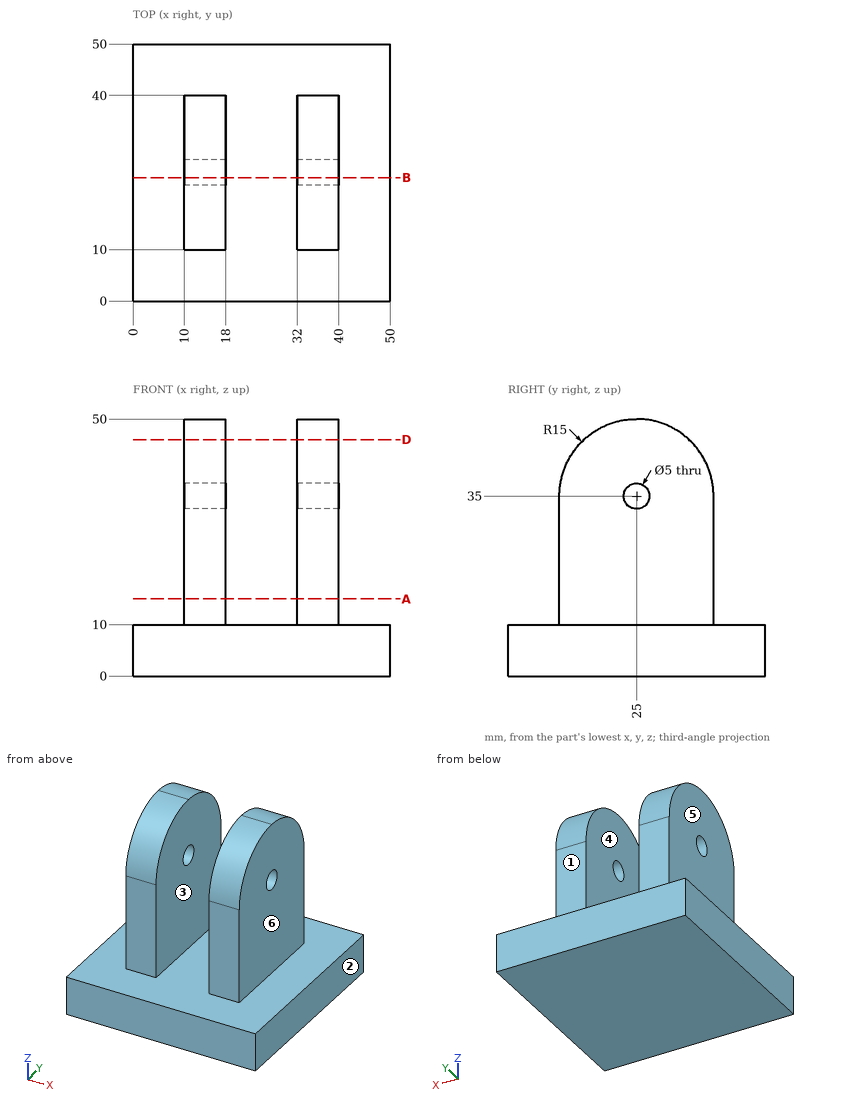
For this review, use the dimensioned drawing (mm, ordinates from the lowest corner) and the shaded views. A direction names the side the tool comes from. Coordinates: 2 decimals unless noted, no trailing zeros. Loops run counter-clockwise (first coordinate to the right, second up) from the corner with the lowest first, then second, coordinate; pieces in that order, holes last. Notation, with made-up numbers: (68.25, 68) -> (99.25, 68) arc R19 ccw to (99.25, 79) -> close; hole circle Ø7 at (-32.75, 37.25). An arc over 180 degrees is marked (long way). Use a Markdown table: item, result. Add a question column.
1. Add section A-A on z = 15. Write out the cut boundary in (x, y), plus the area to 3 significant figures.
2. Clearance check with flat-ended pins moving along their axes: pin 1 Ø6.5 at (x, z) = (12.5, 17.5) entering from +Y; pin 2 Ø2 at (y, z) = (14.5, 25.5) entering from -X; pin 3 Ø9 at (x, z) = (14.5, 26) entering from -Y. State where each tip first meets the part, or that it passes through.
3. Add section D-D on z = 46. Write out the cut boundary in (x, y).
4. Draft analysis for pull direction X (two halves, no side actions). For the marked faces 1, 2 and 3, state which applies: pulls with the +X half, pulls with the -X half, needs draft (parallel to the pull), parting line crosses it, or undercut.
5. Add section B-B on y = 24. Write out the cut boundary in (x, z), plus the area to 3 significant figures.
6. To check wall thickness, follow line 1 (Z direction, x = 15, y = 25); line 2 (X direction, y = 38.5, z = 25.5); line 3 (Z direction, x = 43.5, y = 14.5). State the ranges of each line that lie inside material, in increasing order.
7. Machinability: for the marked faces 4, 5 and 6, which of the approach directions +Z, -Z, +X, -X, +Y, -Y give a long, thin tool a straight path to every point of the face, cutting with its end or side? Answer none if there is none.
Returned:
| question | item | result |
|---|---|---|
| 1 | outline | (10, 10) -> (18, 10) -> (18, 40) -> (10, 40) -> close; (32, 10) -> (40, 10) -> (40, 40) -> (32, 40) -> close |
| 1 | area | 480 mm² |
| 2 | pin 1 | stops at y = 40 |
| 2 | pin 2 | stops at x = 10 |
| 2 | pin 3 | stops at y = 10 |
| 3 | outline | (10, 14.8) -> (18, 14.8) -> (18, 35.2) -> (10, 35.2) -> close; (32, 14.8) -> (40, 14.8) -> (40, 35.2) -> (32, 35.2) -> close |
| 4 | face 1 | needs draft |
| 4 | face 2 | pulls with the +X half |
| 4 | face 3 | undercut |
| 5 | outline | (0, 0) -> (50, 0) -> (50, 10) -> (40, 10) -> (40, 32.71) -> (32, 32.71) -> (32, 10) -> (18, 10) -> (18, 32.71) -> (10, 32.71) -> (10, 10) -> (0, 10) -> close; (10, 37.29) -> (18, 37.29) -> (18, 49.97) -> (10, 49.97) -> close; (32, 37.29) -> (40, 37.29) -> (40, 49.97) -> (32, 49.97) -> close |
| 5 | area | 1,070 mm² |
| 6 | line 1 | z = 0 to 32.5, 37.5 to 50 |
| 6 | line 2 | x = 10 to 18, 32 to 40 |
| 6 | line 3 | z = 0 to 10 |
| 7 | face 4 | +Z, +Y, -Y |
| 7 | face 5 | +Z, -X, +Y, -Y |
| 7 | face 6 | +Z, +X, +Y, -Y |
